Part model, mm, in its own coordinate system. A direction names the side the tool comes from. Coordinates: 2 decimals unless noted, no trailing zeros. Loops run counter-clockwise (first coordinate to the right, second up) from the corner with the lowest first, then second, coordinate; pieces in that order, holes last. Notation, with made-up numbers: (-2.75, -3.75) -> (32.25, -3.75) arc R25 cw to (32.25, 33.25) -> close; hole circle Ø9 at (80, 47.5). An arc over 180 degrees is marked (long way). Use one line per item in the form item = value. Start each with the question number.
(1) Drill centre lines: L1, parallel to X at y = 52, z = 54.5; L2, parallel to Z at x = -46, y = 5.5; L3, parallel to Y at x = -50, z = 130. Where is each one in solid material? Low to high. Write a range as [from, to].
(2) Band-saw the part on B-B on x = 0. Give the cut face in (y, z), then the cut area to 3 significant figures.
(3) Band-saw the part on A-A on y = 29. Give the cut face in (x, z).
(4) 3-axis set-ups, long thin cutter, end or side, ignore diameter. For faces 5 (the flat face through (63.76, 28, 69)), 6 (the flat face through (-60.96, 31, 70)), 7 (the flat face through (-1, -2.8, 38)), 8 (the cylindrical face through (-42.54, 14.51, 1.48)), 9 (the cylindrical face through (-27.31, -1.42, 137.89)): which of +Z, -Z, +X, -X, +Y, -Y reach the whole face in a straight line?
(5) Band-saw the part on C-C on z = 128. Give the cut face in (x, y).
(6) Pin check, flat tips, straight feed: P1, Ø6, axis at y = 1.5, z = 47.5, coming from the -X side; P2, Ø2.5, axis at y = 26, z = 2, coming from the -X side; P3, Ø1.5, axis at x = -47, z = 57, coming from the +Y side. Stop position of each tip, or through.
(7) Mould opens along X. For faces 1 (the flat face through (-1, 12, 0)), 2 (the flat face through (-63.76, 29, 69)), 3 (the cylindrical face through (27.21, -1.42, 137.79)), 4 (the cylindrical face through (65.57, 58.79, 68.87)) say: +X half, -X half, draft (parallel to the pull), parting line (faces both ways), or undercut.
(8) Band-saw the part on D-D on z = 13. Give the cut face in (x, y).
```python
from build123d import *

# Parameters (mm, degrees)
F1_DEPTH = 139.7
F3_DEPTH = 66.301
F4_W     = 126.004966
F4_H     = 65.315597
F5_DEPTH = 3


with BuildPart() as f1:
    # F0 (on Top) → F1 (new body)
    with BuildSketch(Plane.XY):
        with BuildLine():
            Line((60.96, 0), (-60.96, 0))
            Line((-60.96, 0), (-60.96, 63.5))
            Line((-60.96, 63.5), (-70.11, 63.5))
            Line((-70.11, 63.5), (-70.11, 60.7))
            ThreePointArc((-70.11, 60.7), (-65.619872, 58.840128), (-63.76, 54.35))
            Line((-63.76, 54.35), (-63.76, 2.28))
            Line((-63.76, 2.28), (-63.76, -2.8))
            Line((-63.76, -2.8), (-58.68, -2.8))
            Line((-58.68, -2.8), (58.68, -2.8))
            Line((58.68, -2.8), (63.76, -2.8))
            Line((63.76, -2.8), (63.76, 2.28))
            Line((63.76, 2.28), (63.76, 54.35))
            ThreePointArc((63.76, 54.35), (65.619872, 58.840128), (70.11, 60.7))
            Line((70.11, 60.7), (70.11, 63.5))
            Line((70.11, 63.5), (60.96, 63.5))
            Line((60.96, 63.5), (60.96, 0))
        make_face()
        with BuildLine():
            Line((-63.76, -2.8), (-63.76, 2.28))
            ThreePointArc((-63.76, 2.28), (-67.352102, -6.392102), (-58.68, -2.8))
            Line((-58.68, -2.8), (-63.76, -2.8))
        make_face()
        with BuildLine():
            ThreePointArc((58.68, -2.8), (67.352102, -6.392102), (63.76, 2.28))
            Line((63.76, 2.28), (63.76, -2.8))
            Line((63.76, -2.8), (58.68, -2.8))
        make_face()
    extrude(amount=F1_DEPTH)

    # F2 (on face) → F3 (cut, through all)
    with BuildSketch(Plane.XZ.offset(2.8)):
        with BuildLine():
            Line((-25.4, 133.35), (-25.4, 69.85))
            ThreePointArc((-25.4, 69.85), (0, 44.45), (25.4, 69.85))
            Line((25.4, 69.85), (25.4, 133.35))
            ThreePointArc((25.4, 133.35), (27.259872, 137.840128), (31.75, 139.7))
            Line((31.75, 139.7), (41.905578, 139.7))
            Line((41.905578, 139.7), (41.905578, 151.021525))
            Line((41.905578, 151.021525), (-38.783666, 151.021525))
            Line((-38.783666, 151.021525), (-38.783666, 139.7))
            Line((-38.783666, 139.7), (-31.75, 139.7))
            ThreePointArc((-31.75, 139.7), (-27.259872, 137.840128), (-25.4, 133.35))
        make_face()
    extrude(amount=-F3_DEPTH, mode=Mode.SUBTRACT)

    # F4 (on Top) → F5 (join)
    with BuildSketch(Plane.XY):
        with Locations((-0.293547, 30.842202)):
            Rectangle(F4_W, F4_H)
        with BuildLine():
            ThreePointArc((-44.45, 44.45), (-42.590128, 48.940128), (-38.1, 50.8))
            Line((-38.1, 50.8), (38.1, 50.8))
            ThreePointArc((38.1, 50.8), (42.590128, 48.940128), (44.45, 44.45))
            Line((44.45, 44.45), (44.45, 19.05))
            ThreePointArc((44.45, 19.05), (42.590128, 14.559872), (38.1, 12.7))
            Line((38.1, 12.7), (-38.1, 12.7))
            ThreePointArc((-38.1, 12.7), (-42.590128, 14.559872), (-44.45, 19.05))
            Line((-44.45, 19.05), (-44.45, 44.45))
        make_face(mode=Mode.SUBTRACT)
    extrude(amount=F5_DEPTH)


solid = f1.part
```
A:
q1.L1 = [-63.76, -60.96], [60.96, 63.76]
q1.L2 = [0, 3]
q1.L3 = [-2.8, 0]
q2.outline = (-2.8, 0) -> (12.7, 0) -> (12.7, 3) -> (0, 3) -> (0, 44.45) -> (-2.8, 44.45) -> close; (50.8, 0) -> (63.5, 0) -> (63.5, 3) -> (50.8, 3) -> close
q2.area = 201 mm²
q3.outline = (-63.76, 0) -> (-44.45, 0) -> (-44.45, 3) -> (-60.96, 3) -> (-60.96, 139.7) -> (-63.76, 139.7) -> close; (44.45, 0) -> (63.76, 0) -> (63.76, 139.7) -> (60.96, 139.7) -> (60.96, 3) -> (44.45, 3) -> close
q4.face_5 = +Z, -Z, +X
q4.face_6 = +Z, +Y
q4.face_7 = +Z, -Z, -Y
q4.face_8 = +Z, -Z
q4.face_9 = +Z, +Y, -Y
q5.outline = (-70.11, 60.7) arc R6.35 cw to (-63.76, 54.35) -> (-63.76, 2.28) arc R5.08 ccw (long way) to (-58.68, -2.8) -> (-25.4, -2.8) -> (-25.4, 0) -> (-60.96, 0) -> (-60.96, 63.5) -> (-70.11, 63.5) -> close; (25.4, -2.8) -> (58.68, -2.8) arc R5.08 ccw (long way) to (63.76, 2.28) -> (63.76, 54.35) arc R6.35 cw to (70.11, 60.7) -> (70.11, 63.5) -> (60.96, 63.5) -> (60.96, 0) -> (25.4, 0) -> close
q6.P1 = -68.67
q6.P2 = -63.76
q6.P3 = 0
q7.face_1 = draft
q7.face_2 = -X half
q7.face_3 = undercut
q7.face_4 = +X half
q8.outline = (-70.11, 60.7) arc R6.35 cw to (-63.76, 54.35) -> (-63.76, 2.28) arc R5.08 ccw (long way) to (-58.68, -2.8) -> (58.68, -2.8) arc R5.08 ccw (long way) to (63.76, 2.28) -> (63.76, 54.35) arc R6.35 cw to (70.11, 60.7) -> (70.11, 63.5) -> (60.96, 63.5) -> (60.96, 0) -> (-60.96, 0) -> (-60.96, 63.5) -> (-70.11, 63.5) -> close
